Geometry: final body of the model. Coordinates: model frame, mm. Coordinates: 2 decimals unless noted, no trailing zeros. Write each loop counter-clockwise with the first axis right and the second up, starting at its lowest first coordinate (ties: lowest second). Pieces come first, ordered by that corner, then holes. Notation, with made-up numbers: (38.5, 34.25) - (63.5, 34.25) arc R11 ccw to (63.5, 41.25) - close; hole circle Ø9 at (40, 77.25). An arc over 180 degrees is marked (long way). Answer as a JSON object with one key per item and string values. Group by question number.
Item 1: Section A-A on x = 79.5. Return loops of the section in (y, z).
Item 2: Line query: line 1 along X through (y, z) = (-8.5, -5); line 2 along Y through (x, z) = (34, -7.5); line 3 along X through (y, z) = (-4.5, 0.7). Output: solid intervals per line, ascending. Write a range as from..to.
Item 3: Section B-B on z = -5. Return loops of the section in (x, y).
Item 4: First-contact query: pin 1 Ø3 at (x, y) = (-15.5, -5.5) entering from -Z; pin 2 Ø2 at (x, y) = (5, -7.5) entering from -Z; pin 3 Ø4 at (y, z) = (-7, -5.5) entering from -X. Flat tips, straight axial feed; report the tip coordinate or a pass-through.
```python
from build123d import *

# Parameters (mm, degrees)
BASE_FLANGE1_DEPTH            = 1
EDGE_FLANGE1_STRIP_W          = 5
EDGE_FLANGE1_STRIP_H          = 1
EDGE_FLANGE1_STRIP_CUT_DEPTH  = 169
EDGE_FLANGE1_RELIEF_W         = 5.5
EDGE_FLANGE1_RELIEF_H         = 0.5
EDGE_FLANGE1_RELIEF_CUT_DEPTH = 1
EDGE_FLANGE1_DEPTH            = 169
EDGE_FLANGE2_STRIP_W          = 5
EDGE_FLANGE2_STRIP_H          = 1
EDGE_FLANGE2_STRIP_CUT_DEPTH  = 169
EDGE_FLANGE2_DEPTH            = 169
SKETCH12_R                    = 1.5
CUT_EXTRUDE1_DEPTH            = 3
SKETCH13_R                    = 1.5
CUT_EXTRUDE2_DEPTH            = 3


# Sheet-metal steps are written as plain solids
with BuildPart() as part:
    # Sketch1 → Base-Flange1 (new body)
    with BuildSketch(Plane(origin=(0, 0, 0), x_dir=(1, 0, 0), z_dir=(0, 1, 0))):
        Polygon((-84.5, 0), (84.5, 0), (84.5, 10), (-94.5, 10), align=None)
    extrude(amount=-BASE_FLANGE1_DEPTH)

    # Edge-Flange1 strip (across the edge) → Edge-Flange1 strip cut (cut)
    with BuildSketch(Plane(origin=(84.5, -1, 0), x_dir=(0, 0, -1), z_dir=(-1, 0, 0))):
        with Locations((-2, -0.5)):
            Rectangle(EDGE_FLANGE1_STRIP_W, EDGE_FLANGE1_STRIP_H)
    extrude(amount=EDGE_FLANGE1_STRIP_CUT_DEPTH, mode=Mode.SUBTRACT)

    # Edge-Flange1 relief (on the sheet) → Edge-Flange1 relief cut (cut)
    with BuildSketch(Plane(origin=(84.5, -1, -0.5), x_dir=(0, 0, -1), z_dir=(0, -1, 0))):
        with Locations((-2.25, -169.25)):
            Rectangle(EDGE_FLANGE1_RELIEF_W, EDGE_FLANGE1_RELIEF_H)
    extrude(amount=-EDGE_FLANGE1_RELIEF_CUT_DEPTH, mode=Mode.SUBTRACT)

    # Edge-Flange1 section (across the edge) → Edge-Flange1 (add)
    with BuildSketch(Plane(origin=(84.5, -1, 0), x_dir=(0, 0, -1), z_dir=(-1, 0, 0))):
        with BuildLine():
            Line((-1, 0.5), (-1, 7))
            Line((-1, 7), (0, 7))
            Line((0, 7), (0, 0.5))
            ThreePointArc((0, 0.5), (0.146446609, 0.146446609), (0.5, 0))
            Line((0.5, 0), (0.5, -1))
            ThreePointArc((0.5, -1), (-0.560660172, -0.560660172), (-1, 0.5))
        make_face()
    extrude(amount=EDGE_FLANGE1_DEPTH)

    # Edge-Flange2 strip (across the edge) → Edge-Flange2 strip cut (cut)
    with BuildSketch(Plane(origin=(84.5, -8, 0), x_dir=(0, 1, 0), z_dir=(-1, 0, 0))):
        with Locations((-2, -0.5)):
            Rectangle(EDGE_FLANGE2_STRIP_W, EDGE_FLANGE2_STRIP_H)
    extrude(amount=EDGE_FLANGE2_STRIP_CUT_DEPTH, mode=Mode.SUBTRACT)

    # Edge-Flange2 section (across the edge) → Edge-Flange2 (add)
    with BuildSketch(Plane(origin=(84.5, -8, 0), x_dir=(0, 1, 0), z_dir=(-1, 0, 0))):
        with BuildLine():
            Line((-1, 0.5), (-1, 9))
            Line((-1, 9), (0, 9))
            Line((0, 9), (0, 0.5))
            ThreePointArc((0, 0.5), (0.146446609, 0.146446609), (0.5, 0))
            Line((0.5, 0), (0.5, -1))
            ThreePointArc((0.5, -1), (-0.560660172, -0.560660172), (-1, 0.5))
        make_face()
    extrude(amount=EDGE_FLANGE2_DEPTH)

    # Sketch12 → Cut-Extrude1 (cut)
    with BuildSketch(Plane.XZ.offset(9)):
        with Locations(Location((-74.5, -5, 0), (0, 0, 270))):
            Circle(SKETCH12_R)
        with Locations(Location((0, -5, 0), (0, 0, 270))):
            Circle(SKETCH12_R)
        with Locations(Location((74.5, -5, 0), (0, 0, 270))):
            Circle(SKETCH12_R)
    extrude(amount=-CUT_EXTRUDE1_DEPTH, mode=Mode.SUBTRACT)

    # Sketch13 → Cut-Extrude2 (cut)
    with BuildSketch(Plane(origin=(0, 0, 0), x_dir=(-1, 0, 0), z_dir=(0, 0, -1))):
        with Locations(Location((-79.5, -4.5, 0), (0, 0, 90))):
            Circle(SKETCH13_R)
    extrude(amount=-CUT_EXTRUDE2_DEPTH, mode=Mode.SUBTRACT)


solid = part.part
```
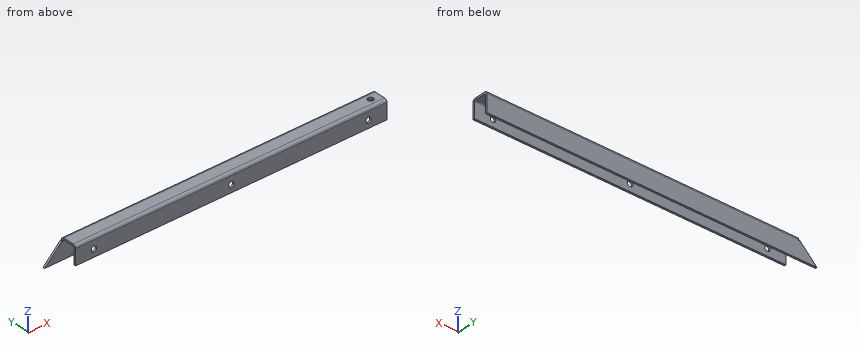
Checks:
{
 "1": {"outline": "(-9, -9) - (-8, -9) - (-8, -0.5) arc R0.5 cw to (-7.5, 0) - (-6, 0) - (-6, 1) - (-7.5, 1) arc R1.5 ccw to (-9, -0.5) - close; (-3, 0) - (-1.5, 0) arc R0.5 cw to (-1, -0.5) - (-1, -10) - (0, -10) - (0, -0.5) arc R1.5 ccw to (-1.5, 1) - (-3, 1) - close"},
 "2": {"line 1": "-84.5..-76, -73..-1.5, 1.5..73, 76..84.5", "line 2": "-9..-8, -1..0", "line 3": "-84.5..78, 81..84.5"},
 "3": {"outline": "(-89.5, -1) - (84.5, -1) - (84.5, 0) - (-89.5, 0) - close; (-84.5, -9) - (-76, -9) - (-76, -8) - (-84.5, -8) - close; (-73, -9) - (-1.5, -9) - (-1.5, -8) - (-73, -8) - close; (1.5, -9) - (73, -9) - (73, -8) - (1.5, -8) - close; (76, -9) - (84.5, -9) - (84.5, -8) - (76, -8) - close"},
 "4": {"pin 1": "z = 0", "pin 2": "z = -9", "pin 3": "x = -84.5"}
}
